Design review of the part built by this model. Coordinates are the model's own, in mm. A direction names the side the tool comes from. Coordinates: 2 decimals unless noted, no trailing zeros. Loops run counter-clockwise (first coordinate to the right, second up) from the corner with the lowest first, then second, coordinate; pieces in that order, holes last. Notation, with made-up numbers: M -6,52 L 33,52 A16 cw 33,74 Z; hole C 59.25,88.5 d11. An arc over 180 degrees is marked long. One line per item, written item: value.
```python
from build123d import *

# Parameters (mm, degrees)
F0_R     = 40
F1_DEPTH = 22
F2_T     = -1.5
F3_R     = 12.5
F4_DEPTH = 6.5
F6_DEPTH = 20.5
F8_DEPTH = 5.5
F9_DEPTH = 0.5


with BuildPart() as f1:
    # F0 (on Right) → F1 (new body)
    with BuildSketch(Plane.YZ):
        Circle(F0_R)
    extrude(amount=F1_DEPTH)

    # F2
    f2_openings = [f1.faces().sort_by_distance(p)[0] for p in [
        (0, 0, 0),
    ]]
    offset(amount=F2_T, openings=f2_openings)

    # F3 (on Right) → F4 (join)
    with BuildSketch(Plane.YZ):
        with Locations((22.9496732003, -13.25)):
            Circle(F3_R)
        with Locations((0, 26.5)):
            Circle(F3_R)
        with Locations((-22.9496732003, -13.25)):
            Circle(F3_R)
    extrude(amount=F4_DEPTH)

    # F5 (on Right) → F6 (cut)
    with BuildSketch(Plane.YZ):
        with BuildLine():
            Line((-23.7566848809, -30.2963681564), (-24.6822700062, -31.4767461365))
            ThreePointArc((-24.6822700062, -31.4767461365), (-16.029318636, -36.6477958964), (-6.3583720579, -39.4914054545))
            Line((-6.3583720579, -39.4914054545), (-6.1199331058, -38.01047775))
            ThreePointArc((-6.1199331058, -38.01047775), (-15.4282191871, -35.2735035503), (-23.7566848809, -30.2963681564))
        make_face()
    extrude(amount=F6_DEPTH, mode=Mode.SUBTRACT)

    # F7 (on face) → F8 (cut)
    with BuildSketch(Plane(origin=(0, 0, 0), x_dir=(0, -1, 0), z_dir=(-1, 0, 0))):
        with BuildLine():
            ThreePointArc((-10.4496732003, -13.25), (-24.0724348464, -0.8005258631), (-35.247978206, -15.4864467321))
            ThreePointArc((-35.247978206, -15.4864467321), (-33.7749907476, -19.5), (-31.0356453874, -22.7824211924))
            ThreePointArc((-31.0356453874, -22.7824211924), (-17.6972762398, -24.5929416894), (-10.4496732003, -13.25))
        make_face()
        with BuildLine():
            ThreePointArc((31.0356453874, -22.7824211924), (33.7749907476, -19.5), (35.247978206, -15.4864467321))
            ThreePointArc((35.247978206, -15.4864467321), (35.3991473372, -14.3727616462), (35.4496732003, -13.25))
            ThreePointArc((35.4496732003, -13.25), (11.6067315109, -7.9976030395), (31.0356453874, -22.7824211924))
        make_face()
        with BuildLine():
            ThreePointArc((4.2123328186, 38.2688679245), (0, 39), (-4.2123328186, 38.2688679245))
            ThreePointArc((-4.2123328186, 38.2688679245), (-7.1970771764, 16.2798199567), (12.5, 26.5))
            ThreePointArc((12.5, 26.5), (10.2201800433, 33.6970771764), (4.2123328186, 38.2688679245))
        make_face()
    extrude(amount=-F8_DEPTH, mode=Mode.SUBTRACT)

    # F9 (cut): a face of the model
    f9_faces = [f1.faces().sort_by_distance(p)[0] for p in [
        (20.5, -0.0988123254, -0.2259144019),
    ]]
    extrude(f9_faces, amount=-F9_DEPTH, mode=Mode.SUBTRACT)


solid = f1.part
```
(1) Mouldability with a two-part tool opening along Z and no side actions: class faces 4 (the flat face through (22, -1, 1)), 5 (the cylindrical face through (10.35, 16.84, 34.62)), 6 (the cylindrical face through (10.85, 21.5, 33.73)) as released by +Z, released by -Z, zero draft, split by the parting line, or undercut.
Reply:
face 4: zero draft
face 5: undercut
face 6: split by the parting line
(2) Tool access review of faces 1 (the flat face through (21, -1, 0)), 2 (the flat face through (0, -15, 36)), 3 (the flat face through (5.5, 0, 27)): name each direction out of +Z, -Z, +X, -X, +Y, -Y from which nothing blocks a thin tool from reaching the whole face with its end or side.
Reply:
face 1: none
face 2: +Z, -Z, -X, +Y, -Y
face 3: -X
(3) We need section C-C on y = 0. State the section outline as (x, z) points, then the cut area to 3 significant figures.
Reply:
outline: M 0,-40 L 22,-40 L 22,40 L 0,40 L 0,39 L 5.5,39 L 5.5,14 L 6.5,14 L 6.5,38.5 L 21,38.5 L 21,-38.5 L 0,-38.5 Z
area: 165 mm2
(4) We need section B-B on x = 2. State the section outline as (y, z) points.
Reply:
outline: M -35.25,-15.49 A38.5 cw -4.21,38.27 A12.5 cw 4.21,38.27 A38.5 cw 35.25,-15.49 A12.5 cw 31.04,-22.78 A38.5 cw -6.12,-38.01 L -6.36,-39.49 A40 ccw long -24.68,-31.48 L -23.76,-30.3 A38.5 cw -31.04,-22.78 A12.5 cw Z
(5) To check wall thickness, follow line 1 along Y through (x, z) = (12.5, 0); line 2 along X through (y, z) = (-22, -17). State the ranges of each line that lie inside material, in increasing order. Write a range as [from, to].
Reply:
line 1: y = [-40, -38.5], [38.5, 40]
line 2: x = [5.5, 6.5], [21, 22]
(6) We need section D-D on z = 20. State the section outline as (x, y) points.
Reply:
outline: M 0,-34.64 L 22,-34.64 L 22,34.64 L 0,34.64 L 0,32.9 L 21,32.9 L 21,-32.9 L 0,-32.9 Z; M 5.5,-10.68 L 6.5,-10.68 L 6.5,10.68 L 5.5,10.68 Z
(7) We need section A-A on z = -7. State the section outline as (x, y) points (3 decimals).
Reply:
outline: M 0,-39.383 L 22,-39.383 L 22,39.383 L 0,39.383 L 0,37.858 L 21,37.858 L 21,-37.858 L 0,-37.858 Z; M 5.5,-33.775 L 6.5,-33.775 L 6.5,-12.124 L 5.5,-12.124 Z; M 5.5,12.124 L 6.5,12.124 L 6.5,33.775 L 5.5,33.775 Z
(8) Insertion check: pin 1 (10 mm diameter, centred on x = 19, z = 16, fed in from -Y); pin 2 (10 mm diameter, centred on x = 15, z = 22.5, fed in from -Y); pin 3 (7.5 mm diameter, centred on y = -5.5, z = 32.5, fed in from -X). Each pin has a flat end and moves straight along its axis. Give the tip position at first contact, or say it passes through.
Reply:
pin 1: stops at y = -38.46
pin 2: stops at y = -35.97
pin 3: stops at x = 5.5
